Source: CAD feature listing. Evaluate the final solid. Frame: model axes, mm. Round coordinates to 2 decimals unless told otherwise and drop trailing zeros. Loops run counter-clockwise (first coordinate to the right, second up) from the corner with the lowest first, then second, coordinate; pieces in that order, holes last. Notation, with made-up numbers: (83.5, 86) -> (136.5, 86) arc R28 cw to (136.5, 107) -> close; hole circle Ø1 at (69.25, 36.5). An arc over 180 degrees is marked (long way). Write item = value, one per line.
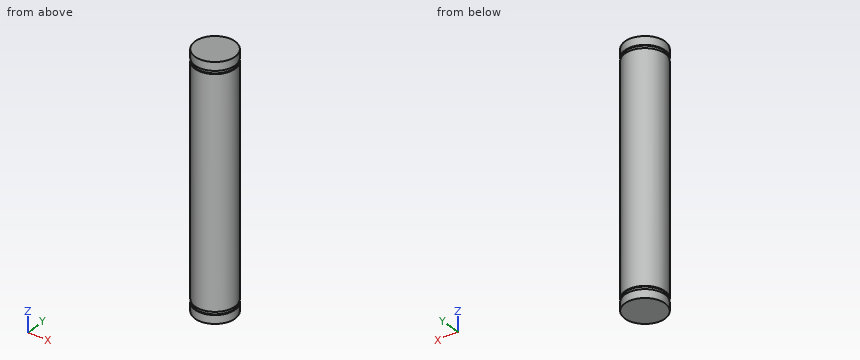
from build123d import *

# Parameters (mm, degrees)
SKETCH1_R           = 4.7625
BOSS_EXTRUDE1_DEPTH = 59.05
SKETCH2_W           = 0.2921
SKETCH2_H           = 0.7366


with BuildPart() as part:
    # Sketch1 → Boss-Extrude1 (new body)
    with BuildSketch(Plane.XY):
        Circle(SKETCH1_R)
    extrude(amount=BOSS_EXTRUDE1_DEPTH)

    # Sketch2 → Cut-Revolve1 (revolve, cut)
    with BuildSketch(Plane(origin=(0, 0, 0), x_dir=(1, 0, 0), z_dir=(0, 1, 0))):
        with Locations((-4.61645, -2.3683)):
            Rectangle(SKETCH2_W, SKETCH2_H)
        with Locations((-4.61645, -56.6817)):
            Rectangle(SKETCH2_W, SKETCH2_H)
    revolve(axis=Axis((0, 0, 0), (0, 0, 1)), mode=Mode.SUBTRACT)


solid = part.part
1. Section query C-C (z = 27.5). Return the cut outline in (x, y) (1 decimal).
Evaluation:
outline = circle Ø9.5 at (0, 0)
2. Line query: probe 1 along Y at (x, z) = (-2.25, 22.5); probe 2 along X at (y, z) = (-3, 6); probe 3 along X at (y, z) = (2.5, 6.5). Output: solid intervals per line, ascending. Write a range as from..to.
Evaluation:
probe_1 = -4.2..4.2
probe_2 = -3.7..3.7
probe_3 = -4.05..4.05
3. Section query B-B (x = 2.75). Return the cut outline in (y, z), then the cut area to 3 significant figures.
Evaluation:
outline = (-3.89, 0) -> (3.89, 0) -> (3.89, 2) -> (3.52, 2) -> (3.52, 2.74) -> (3.89, 2.74) -> (3.89, 56.31) -> (3.52, 56.31) -> (3.52, 57.05) -> (3.89, 57.05) -> (3.89, 59.05) -> (-3.89, 59.05) -> (-3.89, 57.05) -> (-3.52, 57.05) -> (-3.52, 56.31) -> (-3.89, 56.31) -> (-3.89, 2.74) -> (-3.52, 2.74) -> (-3.52, 2) -> (-3.89, 2) -> close
area = 458 mm²
4. Contact query for flat-ended pins moving along their axis: pin 1 Ø5 at (y, z) = (-1.5, 49.5) entering from +X; pin 2 Ø4 at (x, z) = (2.5, 10) entering from -Y. Output: stop coordinate, or through.
Evaluation:
pin_1 = 4.76
pin_2 = -4.74
5. Section query A-A (y = 1). Return the cut outline in (x, z), then the cut area to 3 significant figures.
Evaluation:
outline = (-4.66, 0) -> (4.66, 0) -> (4.66, 2) -> (4.36, 2) -> (4.36, 2.74) -> (4.66, 2.74) -> (4.66, 56.31) -> (4.36, 56.31) -> (4.36, 57.05) -> (4.66, 57.05) -> (4.66, 59.05) -> (-4.66, 59.05) -> (-4.66, 57.05) -> (-4.36, 57.05) -> (-4.36, 56.31) -> (-4.66, 56.31) -> (-4.66, 2.74) -> (-4.36, 2.74) -> (-4.36, 2) -> (-4.66, 2) -> close
area = 549 mm²
